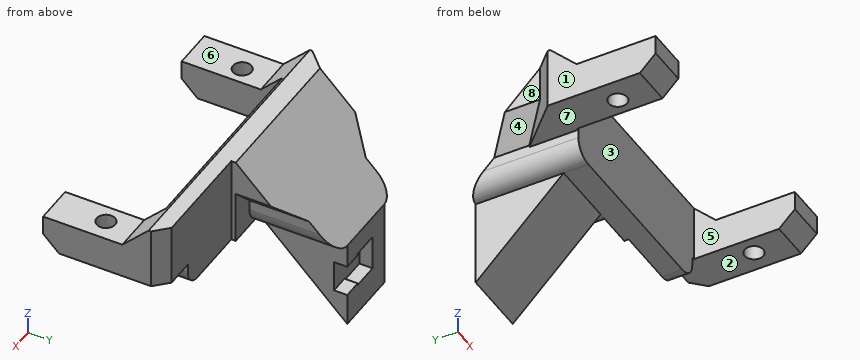
from build123d import *

# Parameters (mm, degrees)
SKETCH1_W             = 23
SKETCH1_H             = 10
BOSS_EXTRUDE1_DEPTH   = 3
SKETCH2_W             = 7
SKETCH2_H             = 3
BOSS_EXTRUDE2_DEPTH   = 4.775
SKETCH3_W             = 7
SKETCH3_H             = 3
BOSS_EXTRUDE3_DEPTH   = 4.775
BOSS_EXTRUDE4_START   = -4.775
BOSS_EXTRUDE4_DEPTH   = 4.775
BOSS_EXTRUDE4_START_2 = 23.130914758
BOSS_EXTRUDE4_2_DEPTH = 4.644085242
SKETCH5_W             = 6.593837141
SKETCH5_H             = 7.601131285
CUT_EXTRUDE1_DEPTH    = 94
CUT_EXTRUDE2_DEPTH    = 94
SKETCH7_R             = 1.05
CUT_EXTRUDE3_DEPTH    = 94
FILLET1_R             = 2
CHAMFER2_SIZE         = 2
CHAMFER3_SIZE         = 2
BOSS_EXTRUDE5_START   = 10
SKETCH8_W             = 3.735996303
SKETCH8_H             = 10
BOSS_EXTRUDE5_DEPTH   = 10
SKETCH10_W            = 1.630996303
SKETCH10_H            = 4
SKETCH10_W_2          = 0.412454303
SKETCH10_H_2          = 2
CUT_EXTRUDE5_DEPTH    = 1.5
SKETCH11_W            = 2.105
SKETCH11_H            = 3.6
CUT_EXTRUDE6_DEPTH    = 1.5
SKETCH14_W            = 12.528007394
SKETCH14_H            = 0.5
CUT_EXTRUDE9_DEPTH    = 14
CHAMFER4_SIZE         = 10
CHAMFER5_SIZE         = 10
CHAMFER6_SIZE         = 3
SKETCH12_W            = 32.55
SKETCH12_H            = 6
CUT_EXTRUDE7_DEPTH    = 3
SKETCH13_W            = 32.55
SKETCH13_H            = 3
CUT_EXTRUDE8_DEPTH    = 3
CHAMFER7_SIZE         = 3


# Read off the part's stored shape, not the designer's step: Boss-Extrude4
# Some blends are built 0.0001 mm under size
with BuildPart() as part:
    # Sketch1 → Boss-Extrude1 (new body)
    with BuildSketch(Plane(origin=(0, 0, 0), x_dir=(1, 0, 0), z_dir=(0, 1, 0))):
        with Locations((11.5, 5)):
            Rectangle(SKETCH1_W, SKETCH1_H)
    extrude(amount=BOSS_EXTRUDE1_DEPTH)

    # Sketch2 → Boss-Extrude2 (add)
    with BuildSketch(Plane(origin=(23, 0, 0), x_dir=(0, 0, -1), z_dir=(1, 0, 0))):
        with Locations((3.5, 1.5)):
            Rectangle(SKETCH2_W, SKETCH2_H)
    extrude(amount=BOSS_EXTRUDE2_DEPTH)

    # Sketch3 → Boss-Extrude3 (add)
    with BuildSketch(Plane.ZY):
        with Locations((-3.5, 1.5)):
            Rectangle(SKETCH3_W, SKETCH3_H)
    extrude(amount=BOSS_EXTRUDE3_DEPTH)

    # Boss-Extrude4 outline → Boss-Extrude4 (add)
    with BuildSketch(Plane.YZ.offset(BOSS_EXTRUDE4_START)):
        Polygon((0, 0), (-16.48071009, 0), (-9.48071009, -7), (0, -7), align=None)
    extrude(amount=BOSS_EXTRUDE4_DEPTH)

    # Boss-Extrude4 2 outline → Boss-Extrude4 2 (add)
    with BuildSketch(Plane.YZ.offset(BOSS_EXTRUDE4_START_2)):
        Polygon((0, 0), (-16.48071009, 0), (-9.48071009, -7), (0, -7), align=None)
    extrude(amount=BOSS_EXTRUDE4_2_DEPTH)

    # Sketch5 → Cut-Extrude1 (cut)
    with BuildSketch(Plane.ZY.offset(4.775)):
        with Locations((-3.296918571, -15.081275732)):
            Rectangle(SKETCH5_W, SKETCH5_H)
    extrude(amount=-CUT_EXTRUDE1_DEPTH, mode=Mode.SUBTRACT)

    # Sketch6 → Cut-Extrude2 (cut)
    with BuildSketch(Plane.XY):
        Polygon((23.330914758, 0.2), (-0.2, 0.2), (-0.2, -11.28071009), (0, -11.28071009), (0, 0), (23.130914758, 0), (23.130914758, -11.28071009), (23.330914758, -11.28071009), align=None)
    extrude(amount=-CUT_EXTRUDE2_DEPTH, mode=Mode.SUBTRACT)

    # Sketch7 → Cut-Extrude3 (cut)
    with BuildSketch(Plane(origin=(0, 0, -7), x_dir=(-1, 0, 0), z_dir=(0, 0, -1))):
        with Locations((2.119085242, -5.48071009)):
            Circle(SKETCH7_R)
        with Locations((-25.380914758, -5.48071009)):
            Circle(SKETCH7_R)
    extrude(amount=-CUT_EXTRUDE3_DEPTH, mode=Mode.SUBTRACT)

    # Fillet1
    fillet1_edges = [part.edges().sort_by_distance(p)[0] for p in [
        (0, 1.6, -10),
        (23, 1.6, -10),
    ]]
    fillet(fillet1_edges, radius=FILLET1_R)

    # Chamfer2
    chamfer2_edges = [part.edges().sort_by_distance(p)[0] for p in [
        (27.775, 3, -3.5),
        (-4.775, 3, -3.5),
    ]]
    chamfer(chamfer2_edges, length=CHAMFER2_SIZE)

    # Chamfer3
    chamfer3_edges = [part.edges().sort_by_distance(p)[0] for p in [
        (25.552957379, -11.28071009, 0),
    ]]
    chamfer(chamfer3_edges, length=CHAMFER3_SIZE)

    # Sketch8 → Boss-Extrude5 (add)
    with BuildSketch(Plane(origin=(0, 3, 0), x_dir=(1, 0, 0), z_dir=(0, 1, 0)).offset(BOSS_EXTRUDE5_START)):
        with BuildLine():
            Line((9.471992606, 10), (5.735996303, 10))
            Line((5.735996303, 10), (5.735996303, 0))
            Line((5.735996303, 0), (14.246992606, 0))
            Line((14.246992606, 0), (14.246992606, 7))
            Line((14.246992606, 7), (11.471992606, 7))
            Line((11.471992606, 7), (11.471992606, 8))
            ThreePointArc((11.471992606, 8), (10.886206168, 9.414213562), (9.471992606, 10))
        make_face()
        with BuildLine():
            Line((5.735996303, 0), (5.735996303, 10))
            Line((5.735996303, 10), (2, 10))
            ThreePointArc((2, 10), (0.585786438, 9.414213562), (0, 8))
            Line((0, 8), (0, 7))
            Line((0, 7), (-2.775, 7))
            Line((-2.775, 7), (-2.775, 0))
            Line((-2.775, 0), (5.735996303, 0))
        make_face()
        with Locations((3.867998152, 15)):
            Rectangle(SKETCH8_W, SKETCH8_H)
        with Locations((7.603994455, 15)):
            Rectangle(SKETCH8_W, SKETCH8_H)
    extrude(amount=-BOSS_EXTRUDE5_DEPTH)

    # Sketch10 → Cut-Extrude5 (cut)
    with BuildSketch(Plane(origin=(0, 13, 0), x_dir=(1, 0, 0), z_dir=(0, 1, 0))):
        with Locations((6.551494455, 14.49800095)):
            Rectangle(SKETCH10_W, SKETCH10_H)
        with Locations((4.573219758, 13.49800095)):
            Rectangle(SKETCH10_W_2, SKETCH10_H_2)
        with Locations((4.573219758, 15.49800095)):
            Rectangle(SKETCH10_W_2, SKETCH10_H_2)
        Polygon((5.735996303, 16.49800095), (4.779446909, 16.49800095), (4.779446909, 14.49800095), (4.779446909, 12.49800095), (5.735996303, 12.49800095), align=None)
    extrude(amount=-CUT_EXTRUDE5_DEPTH, mode=Mode.SUBTRACT)

    # Sketch11 → Cut-Extrude6 (cut)
    with BuildSketch(Plane(origin=(0, 13, 0), x_dir=(1, 0, 0), z_dir=(0, 1, 0))):
        with Locations((8.419492606, 14.49800095)):
            Rectangle(SKETCH11_W, SKETCH11_H)
    extrude(amount=-CUT_EXTRUDE6_DEPTH, mode=Mode.SUBTRACT)

    # Sketch14 → Cut-Extrude9 (cut)
    with BuildSketch(Plane.XY):
        with Locations((20.510996303, 2.75)):
            Rectangle(SKETCH14_W, SKETCH14_H)
    extrude(amount=-CUT_EXTRUDE9_DEPTH, mode=Mode.SUBTRACT)

    # Chamfer4
    chamfer4_edges = [part.edges().sort_by_distance(p)[0] for p in [
        (5.735996303, 3, -20),
    ]]
    chamfer(chamfer4_edges, length=CHAMFER4_SIZE - 0.0001)  # a hair under: the kernel refuses the full size

    # Chamfer5
    chamfer5_edges = [part.edges().sort_by_distance(p)[0] for p in [
        (5.735996303, 13, 0),
    ]]
    chamfer(chamfer5_edges, length=CHAMFER5_SIZE)

    # Chamfer6
    # the kernel refuses this chamfer: 3 mm, written as the material it takes off along each edge
    with BuildSketch(Plane(origin=(-2.775, 17.715048964, -7), x_dir=(0.9996219169112968, 0, -0.02749587661058649), z_dir=(0, -1, 0))) as chamfer6_piece_1_section:
        Polygon((CHAMFER6_SIZE * 0.999621916911, CHAMFER6_SIZE * 0.0274958766106), (-CHAMFER6_SIZE * 0.0274958766106, CHAMFER6_SIZE * 0.999621916911), (0, 0), align=None)
    chamfer6_piece_1 = extrude(amount=22.430097928, mode=Mode.PRIVATE)
    chamfer6_piece_1 = split(chamfer6_piece_1, bisect_by=Plane(origin=(0, 7.74942321, -6.834490118), z_dir=(-1, 0, 0)), keep=Keep.TOP, mode=Mode.PRIVATE)
    chamfer6_piece_1 = split(chamfer6_piece_1, bisect_by=Plane(origin=(0.931889756, 6.706889756, -6.834490118), z_dir=(-0.7071067811865476, 0.7071067811865476, 0)), keep=Keep.TOP, mode=Mode.PRIVATE)
    add(chamfer6_piece_1, mode=Mode.SUBTRACT)
    with BuildSketch(Plane(origin=(14.246992606, 17.715048964, -7), x_dir=(-0.9996219169112969, 0, -0.027495876610586497), z_dir=(0, -1, 0))) as chamfer6_piece_2_section:
        Polygon((CHAMFER6_SIZE * 0.999621916911, -CHAMFER6_SIZE * 0.0274958766106), (-CHAMFER6_SIZE * 0.0274958766106, -CHAMFER6_SIZE * 0.999621916911), (0, 0), align=None)
    chamfer6_piece_2 = extrude(amount=14.715048964, mode=Mode.PRIVATE)
    chamfer6_piece_2 = split(chamfer6_piece_2, bisect_by=Plane(origin=(11.471992606, 6.038915357, -6.077830715), z_dir=(1, 0, 0)), keep=Keep.TOP, mode=Mode.PRIVATE)
    add(chamfer6_piece_2, mode=Mode.SUBTRACT)

    # Sketch12 → Cut-Extrude7 (cut)
    with BuildSketch(Plane.XY):
        with Locations((11.5, -5.28071009)):
            Rectangle(SKETCH12_W, SKETCH12_H)
    extrude(amount=-CUT_EXTRUDE7_DEPTH, mode=Mode.SUBTRACT)

    # Sketch13 → Cut-Extrude8 (cut)
    with BuildSketch(Plane(origin=(0, -8.28071009, 0), x_dir=(1, 0, 0), z_dir=(0, 1, 0))):
        with Locations((11.5, 1.5)):
            Rectangle(SKETCH13_W, SKETCH13_H)
    extrude(amount=-CUT_EXTRUDE8_DEPTH, mode=Mode.SUBTRACT)

    # Chamfer7
    chamfer7_edges = [part.edges().sort_by_distance(p)[0] for p in [
        (25.552957379, -2.28071009, 0),
    ]]
    chamfer(chamfer7_edges, length=CHAMFER7_SIZE - 0.0001)  # a hair under: the kernel refuses the full size


solid = part.part
The model under review builds one solid part; all positions refer to its coordinate system, in mm. Face numbers are marked on the shaded views. A direction names the side the tool comes from. Round coordinates to 2 decimals unless told otherwise and drop trailing zeros. Order: outer loops, then holes, each group sorted by start corner. A loop starts at its lowest first (then second) coordinate and runs counter-clockwise, first axis right, second up. Notation, with made-up numbers: (-12, 65.25) -> (32, 65.25) arc R8 ccw to (32, 70.25) -> close; hole circle Ø10 at (89, 88). An arc over 180 degrees is marked (long way). Write item = value, one per line. Start each with the question number.
Item 1: Consider section D-D on x = 11. Write out the cut boundary in (y, z), plus the area to 3 significant figures.
Item 2: Clearance check with flat-ended pins moving along their axes: pin 1 Ø0.5 at (y, z) = (2, -7.5) entering from +X; pin 2 Ø5 at (x, z) = (19.5, -3.5) entering from +Y; pin 3 Ø8 at (x, y) = (3, -5.5) entering from -Z. State where each tip first meets the part, or that it passes through.
Item 3: For line 1 along Y through (x, z) = (19.5, -2.5); line 2 along X through (y, z) = (10.5, -13.75); line 3 along Z through (x, y) = (4, 6.5), list the stretches that pass through material, from the lowest coordinate up.
Item 4: Consider section C-C on z = -15.75. Write out the cut boundary in (x, y).
Item 5: Mouldability with a two-part tool opening along X and no side actions: class the marked faces 1, 2 and 3 as released by +X, released by -X, zero draft, split by the parting line, or undercut.
Item 6: Consider section B-B on x = 15. Write out the cut boundary in (y, z).
Item 7: For the marked faces 4, 5, 6, 7 and 8, list the 3-axis set-ups (+Z, -Z, +X, -X, +Y, -Y) from which the entire face can be reached by the end or side of a thin tool; tool diameter is ignored.
Conclusion:
q1.outline = (0.2, -10) -> (3, -10) -> (3, -9.29) -> (12.29, -9.29) -> (3, 0) -> (0.72, 0) -> (0.2, -0.52) -> close
q1.area = 71.0 mm2
q2.pin_1 = 23
q2.pin_2 = 2.5
q2.pin_3 = -7
q3.line_1 = 0.2 to 2.5
q3.line_2 = 2 to 9.47
q3.line_3 = -13.5 to -3.5
q4.outline = (2, 8.75) -> (9.47, 8.75) -> (9.47, 11.5) -> (4.37, 11.5) -> (4.37, 13) -> (2, 13) -> close
q5.face_1 = released by -X
q5.face_2 = zero draft
q5.face_3 = undercut
q6.outline = (0.2, -10) -> (2.5, -10) -> (2.5, 0) -> (0.72, 0) -> (0.2, -0.52) -> close
q7.face_4 = -Z, -X, +Y
q7.face_5 = +Z, -Z, -Y
q7.face_6 = +Z, +X, -X, -Y
q7.face_7 = -Z, -X, +Y, -Y
q7.face_8 = +Z, -Z, -X, +Y
